Here's how the part is built. I have some questions about the finished solid (model axes, mm). A direction names the side the tool comes from. Coordinates: 2 decimals unless noted, no trailing zeros. Write each loop counter-clockwise with the first axis right and the second up, starting at its lowest first coordinate (ties: lowest second). Pieces come first, ordered by that corner, then holes.
```python
from build123d import *

# Parameters (mm, degrees)
F1_DEPTH = 21.6916
F3_DEPTH = 2


with BuildPart() as f1:
    # F0 (on Top) → F1 (new body)
    with BuildSketch(Plane.XY):
        Polygon((31.633887, 76.3081), (25.42258, 87.0664), (11.845265, 87.0664), (5.633957, 76.3081), (-6.788658, 76.3081), (-13.577315, 64.5498), (-7.366008, 53.7915), (-13.577315, 43.0332), (-7.366008, 32.2749), (-13.577315, 21.5166), (-7.366008, 10.7583), (-13.577315, 0), (-6.788658, -11.7583), (6.788658, -11.7583), (12.999965, -1), (24.267879, -1), (30.479187, -11.7583), (44.056502, -11.7583), (50.267809, -1), (62.690424, -1), (69.479082, 10.7583), (63.267775, 21.5166), (69.479082, 32.2749), (63.267775, 43.0332), (69.479082, 53.7915), (63.267775, 64.5498), (69.479082, 75.3081), (62.690424, 87.0664), (49.113109, 87.0664), (42.901802, 76.3081), align=None)
        Polygon((-5.633957, 9.7583), (5.633957, 9.7583), (11.267914, 0), (5.633957, -9.7583), (-5.633957, -9.7583), (-11.267914, 0), align=None, mode=Mode.SUBTRACT)
        Polygon((12.999965, 20.5166), (24.267879, 20.5166), (29.901836, 10.7583), (24.267879, 1), (12.999965, 1), (7.366008, 10.7583), align=None, mode=Mode.SUBTRACT)
        Polygon((11.267914, 21.5166), (5.633957, 11.7583), (-5.633957, 11.7583), (-11.267914, 21.5166), (-5.633957, 31.2749), (5.633957, 31.2749), align=None, mode=Mode.SUBTRACT)
        Polygon((24.267879, 22.5166), (12.999965, 22.5166), (7.366008, 32.2749), (12.999965, 42.0332), (24.267879, 42.0332), (29.901836, 32.2749), align=None, mode=Mode.SUBTRACT)
        Polygon((48.535759, 0), (42.901802, -9.7583), (31.633887, -9.7583), (25.99993, 0), (31.633887, 9.7583), (42.901802, 9.7583), align=None, mode=Mode.SUBTRACT)
        Polygon((61.535724, 1), (50.267809, 1), (44.633852, 10.7583), (50.267809, 20.5166), (61.535724, 20.5166), (67.169681, 10.7583), align=None, mode=Mode.SUBTRACT)
        Polygon((25.99993, 21.5166), (31.633887, 31.2749), (42.901802, 31.2749), (48.535759, 21.5166), (42.901802, 11.7583), (31.633887, 11.7583), align=None, mode=Mode.SUBTRACT)
        Polygon((67.169681, 32.2749), (61.535724, 22.5166), (50.267809, 22.5166), (44.633852, 32.2749), (50.267809, 42.0332), (61.535724, 42.0332), align=None, mode=Mode.SUBTRACT)
        Polygon((11.267914, 43.0332), (5.633957, 33.2749), (-5.633957, 33.2749), (-11.267914, 43.0332), (-5.633957, 52.7915), (5.633957, 52.7915), align=None, mode=Mode.SUBTRACT)
        Polygon((24.267879, 44.0332), (12.999965, 44.0332), (7.366008, 53.7915), (12.999965, 63.5498), (24.267879, 63.5498), (29.901836, 53.7915), align=None, mode=Mode.SUBTRACT)
        Polygon((11.267914, 64.5498), (5.633957, 54.7915), (-5.633957, 54.7915), (-11.267914, 64.5498), (-5.633957, 74.3081), (5.633957, 74.3081), align=None, mode=Mode.SUBTRACT)
        Polygon((24.267879, 65.5498), (12.999965, 65.5498), (7.366008, 75.3081), (12.999965, 85.0664), (24.267879, 85.0664), (29.901836, 75.3081), align=None, mode=Mode.SUBTRACT)
        Polygon((25.99993, 43.0332), (31.633887, 52.7915), (42.901802, 52.7915), (48.535759, 43.0332), (42.901802, 33.2749), (31.633887, 33.2749), align=None, mode=Mode.SUBTRACT)
        Polygon((50.267809, 63.5498), (61.535724, 63.5498), (67.169681, 53.7915), (61.535724, 44.0332), (50.267809, 44.0332), (44.633852, 53.7915), align=None, mode=Mode.SUBTRACT)
        Polygon((31.633887, 54.7915), (25.99993, 64.5498), (31.633887, 74.3081), (42.901802, 74.3081), (48.535759, 64.5498), (42.901802, 54.7915), align=None, mode=Mode.SUBTRACT)
        Polygon((44.633852, 75.3081), (50.267809, 85.0664), (61.535724, 85.0664), (67.169681, 75.3081), (61.535724, 65.5498), (50.267809, 65.5498), align=None, mode=Mode.SUBTRACT)
    extrude(amount=F1_DEPTH)

    # F2 (on face) → F3 (join)
    with BuildSketch(Plane(origin=(0, 0, 0), x_dir=(1, 0, 0), z_dir=(0, 0, -1))):
        Polygon((49.113109, -87.0664), (62.690424, -87.0664), (69.479082, -75.3081), (63.267775, -64.5498), (69.479082, -53.7915), (63.267775, -43.0332), (69.479082, -32.2749), (63.267775, -21.5166), (69.479082, -10.7583), (62.690424, 1), (50.267809, 1), (44.056502, 11.7583), (30.479187, 11.7583), (24.267879, 1), (12.999965, 1), (6.788658, 11.7583), (-6.788658, 11.7583), (-13.577315, 0), (-7.366008, -10.7583), (-13.577315, -21.5166), (-7.366008, -32.2749), (-13.577315, -43.0332), (-7.366008, -53.7915), (-13.577315, -64.5498), (-6.788658, -76.3081), (5.633957, -76.3081), (11.845265, -87.0664), (25.42258, -87.0664), (31.633887, -76.3081), (42.901802, -76.3081), align=None)
    extrude(amount=F3_DEPTH)


solid = f1.part
```
1) Imagine slicing it at B-B on y = 78.5. Please give me the cut outline in (x, z).
Values follow:
outline: (6.9, -2) - (30.37, -2) - (30.37, 21.69) - (28.06, 21.69) - (28.06, 0) - (9.21, 0) - (9.21, 21.69) - (6.9, 21.69) - close; (44.17, -2) - (67.64, -2) - (67.64, 21.69) - (65.33, 21.69) - (65.33, 0) - (46.48, 0) - (46.48, 21.69) - (44.17, 21.69) - close
2) Will these pins go through, and if not, where does the flat tip stop? pin 1 (10 mm diameter, centred on x = 16, y = 37, fed in from +Z); pin 2 (12 mm diameter, centred on x = 57, z = 19, fed in from -Y); pin 3 (2 mm diameter, centred on y = 61, z = 5, fed in from +X).
Values follow:
pin 1: stops at z = 0
pin 2: stops at y = -1
pin 3: stops at x = 65.89
3) On a 3-axis mill with a long thin cutter (end or side, diameter ignored), from which of +Z, -Z, +X, -X, +Y, -Y can I reach the whole of each face in a straight line? I mean faces 4 (the face through (-1, 76.308, 10)), 5 (the face through (0, 54.792, 11)), 6 (the face through (28.485, 81.763, 10.012)), 7 (the face through (66.33, 59.246, 10.012)). Say none if no direction works.
Values follow:
face 4: +Z, -Z, -X, +Y
face 5: +Z
face 6: +Z, -Z, +Y
face 7: +Z, -Z, +X
4) Imagine slicing it at A-A on x = 3. Please give me the cut outline in (y, z), then the cut area to 3 significant figures.
Values follow:
outline: (-11.76, -2) - (76.31, -2) - (76.31, 21.69) - (74.31, 21.69) - (74.31, 0) - (54.79, 0) - (54.79, 21.69) - (52.79, 21.69) - (52.79, 0) - (33.27, 0) - (33.27, 21.69) - (31.27, 21.69) - (31.27, 0) - (11.76, 0) - (11.76, 21.69) - (9.76, 21.69) - (9.76, 0) - (-9.76, 0) - (-9.76, 21.69) - (-11.76, 21.69) - close
area: 393 mm2
5) Imagine slicing it at C-C on z = 6.75. Count the separate pieces of the cut face and the enclosed holes in it, then the cut area to 3 significant figures.
Values follow:
separate pieces: 1
enclosed holes: 16
area: 1,510 mm2
6) We'd pull the mould along X, two halves only. Please class faces 1 (the face through (-10.43, 37.58, 10.01)), 2 (the face through (66.42, 48.49, 10.01)), 3 (the face through (18, 11, 0)): pulls with the +X half, pulls with the -X half, needs draft (parallel to the pull), parting line crosses it, or undercut.
Values follow:
face 1: pulls with the -X half
face 2: pulls with the +X half
face 3: undercut
7) I need wall thicknesses on probe 1 along Y at (x, z) = (60, 9); probe 2 along Y at (x, z) = (38.5, 3.75); probe 3 along X at (y, z) = (49, 5.5). Which ranges of each line are inside material? Lowest first, please.
Values follow:
probe 1: y = -1 to 1, 20.52 to 22.52, 42.03 to 44.03, 63.55 to 65.55, 85.07 to 87.07
probe 2: y = -11.76 to -9.76, 9.76 to 11.76, 31.27 to 33.27, 52.79 to 54.79, 74.31 to 76.31
probe 3: x = -10.13 to -7.82, 7.82 to 10.13, 27.14 to 29.44, 45.09 to 47.4, 64.4 to 66.71
